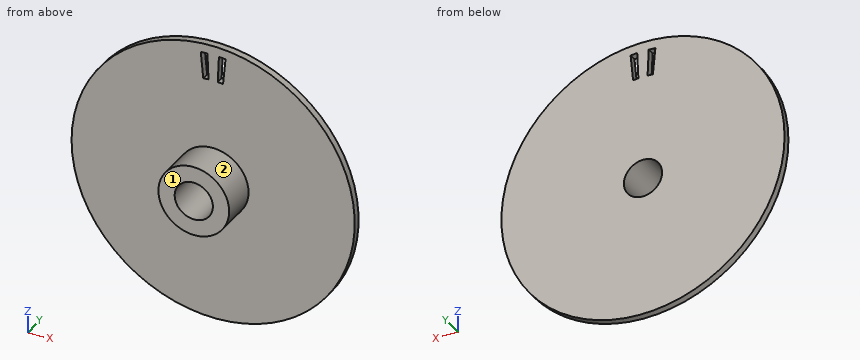
Autodesk Inventor part; units mm, degrees
ref_plane "YZ Plane" through (0, 0, 0) normal (1, 0, 0) x (0, 1, 0)
ref_plane "XZ Plane" through (0, 0, 0) normal (0, 1, 0) x (-1, 0, 0)
ref_plane "XY Plane" through (0, 0, 0) normal (0, 0, 1) x (1, 0, 0)
sketch "Sketch1" plane through (0, 0, 0) normal (0, 1, 0) x (-1, 0, 0)
  circle A0 centre (0, 0) radius 20
  line L0 (0, 0) -> (20, 0)
  circle A1 centre (0, 0) radius 2.7
  dimension "d1" = 40
  dimension "d6" = 5.4
extrude "Extrusion1" add sketch "Sketch1" along normal blind 6
sketch "Sketch2" plane through (0, 0, 0) normal (0, -1, 0) x (1, 0, 0)
  circle A0 centre (0, 0) radius 2.7
  circle A1 centre (0, 0) radius 20
  circle A2 centre (0, 0) radius 5
  circle A3 centre (0, 0) radius 11.1111
  dimension "d7" = 10
extrude "Extrusion2" cut sketch "Sketch2" against normal blind 5 contours A1 | A3
sketch "Sketch3" plane through (0, 6, 0) normal (0, 1, 0) x (1, 0, 0)
  circle A0 centre (0, 0) radius 2.7
  circle A1 centre (0, 0) radius 20
  line L0 (0, 0) -> (0, -20)
  circle A2 centre (0, 0) radius 20
  line L1 (2.4, -13.5) -> (2.4, -20)
  line L2 (2.4, -20) -> (-2.4, -20)
  line L3 (-2.4, -20) -> (-2.4, -13.5)
  line L4 (-2.4, -13.5) -> (2.4, -13.5)
  line L5 (2.4, -13.5) -> (-2.4, -20) construction
  line L6 (2.4, -20) -> (-2.4, -13.5) construction
  line L7 (0.25, -18.6) -> (1.75, -18.6)
  line L8 (1.75, -18.6) -> (1.75, -14.9)
  line L9 (1.75, -14.9) -> (0.25, -14.9)
  line L10 (0.25, -14.9) -> (0.25, -18.6)
  line L11 (-0.25, -18.6) -> (-1.75, -18.6)
  line L12 (-1.75, -18.6) -> (-1.75, -14.9)
  line L13 (-1.75, -14.9) -> (-0.25, -14.9)
  line L14 (-0.25, -14.9) -> (-0.25, -18.6)
  arc A3 (-0.8149, -18.6644) -> (-1.75, -18.6) centre (0, 0) ccw
  arc A4 (-0.65, -14.8879) -> (-1.3959, -14.8366) centre (0, 0) ccw
  line L15 (0, 0) -> (-0.65, -14.8879)
  line L16 (0, 0) -> (0.65, -14.8879)
  line L17 (0, 0) -> (-1.3959, -14.8366)
  line L18 (0, 0) -> (1.3959, -14.8366)
  arc A5 (-1.3959, -14.8366) -> (-0.65, -14.8879) centre (0, 0) ccw
  arc A6 (-1.3886, -18.6305) -> (-0.8149, -18.6644) centre (0, 0) ccw
  arc A7 (-1.75, -18.6) -> (-1.3886, -18.6305) centre (0, 0) ccw
  line L19 (-0.65, -14.8879) -> (-0.8149, -18.6644)
  line L20 (-1.3959, -14.8366) -> (-1.75, -18.6)
  line L21 (1.3959, -14.8366) -> (1.75, -18.6)
  line L22 (0.65, -14.8879) -> (0.8149, -18.6644)
  point P0 (0, -16.75)
  dimension "d10" = 0
  dimension "d11" = 4.8
  dimension "d12" = 6.5
  dimension "d13" = 1.5
  dimension "d14" = 3.7
  dimension "d17" = 1.4
  dimension "d40" = 2
  dimension "d41" = 0.25
  dimension "d76" = 5
  dimension "d77" = 2.5
extrude "Extrusion4" cut sketch "Sketch3" against normal blind 10 contours A5 L19 L13 L20 | L21 L9 L22 A4 | L13 L19 L11 L20 | L21 L7 L22 L9 | L11 L19 A6 A7 | A3 L22 L7
equation "\"d17\" = -0.5 * d14 + 0.5 * d12"
equation "\"d41\" = -0.5 * d13 + 0.5 * d40"
equation "\"d77\" = 0.5 * d76"
properties part number "SmallPositionDisk"
The model under review builds one solid part; all positions refer to its coordinate system, in mm. Face numbers are marked on the shaded views. A direction names the side the tool comes from. Round coordinates to 2 decimals unless told otherwise and drop trailing zeros. Loops run counter-clockwise (first coordinate to the right, second up) from the corner with the lowest first, then second, coordinate; pieces in that order, holes last. Notation, with made-up numbers: (26.5, 2.25) - (57.5, 2.25) arc R19 cw to (57.5, 10.25) - close; hole circle Ø10 at (21.25, 89). An arc over 180 degrees is marked (long way). Write each question's results on one line, items separated by ' | '. Start each with the question number.
Q1. Tool access review of the marked faces 1 and 2: name each direction out of +Z, -Z, +X, -X, +Y, -Y from which nothing blocks a thin tool from reaching the whole face with its end or side.
Q2. Take a section at D-D on x = -4.5. Give the boundary of the cut face in (y, z).
Q3. Take a section at A-A on z = 0. Give the boundary of the cut face in (x, y).
Q4. Wall thickness on line 1 along Z through (x, y) = (0, 1.55); line 2 along Y through (x, z) = (16, 0.5); line 3 along Z through (x, y) = (2, 1.5): over which ranges is each line inside the solid? List them lowest first. Write a range as [from, to].
Q5. Take a section at C-C on y = 1.9. Give the boundary of the cut face in (x, z).
Q6. Take a section at B-B on x = 0. Give the boundary of the cut face in (y, z), plus the area to 3 significant figures.
Data:
1) face 1: +Z, -Z, +X, -X, -Y | face 2: -Y
2) outline: (0, -2.18) - (5, -2.18) - (5, -19.49) - (6, -19.49) - (6, 19.49) - (5, 19.49) - (5, 2.18) - (0, 2.18) - close
3) outline: (-20, 5) - (-5, 5) - (-5, 0) - (-2.7, 0) - (-2.7, 6) - (-20, 6) - close; (2.7, 0) - (5, 0) - (5, 5) - (20, 5) - (20, 6) - (2.7, 6) - close
4) line 1: z = [-5, -2.7], [2.7, 5] | line 2: y = [5, 6] | line 3: z = [-4.58, -1.81], [1.81, 4.58]
5) outline: circle Ø10 at (0, 0); hole circle Ø5.4 at (0, 0)
6) outline: (0, -5) - (5, -5) - (5, -20) - (6, -20) - (6, -2.7) - (0, -2.7) - close; (0, 2.7) - (6, 2.7) - (6, 20) - (5, 20) - (5, 5) - (0, 5) - close | area: 57.6 mm²
